The figure shows three views and two pictorial views of one solid part (mm, origin at its lowest corner). Answer the questions. A direction names the side the tool comes from. Coordinates: 2 decimals unless noted, no trailing zeros. Write each loop counter-clockwise with the first axis right and the second up, starting at its lowest first coordinate (ties: lowest second). Pieces come first, ordered by that corner, then holes. Notation, with made-up numbers: M 83.5,6 L 125.5,6 A26 cw 125.5,35 Z; hole C 47.25,63 d2. An arc over 180 degrees is marked long. Answer as CSV lines item,"result".
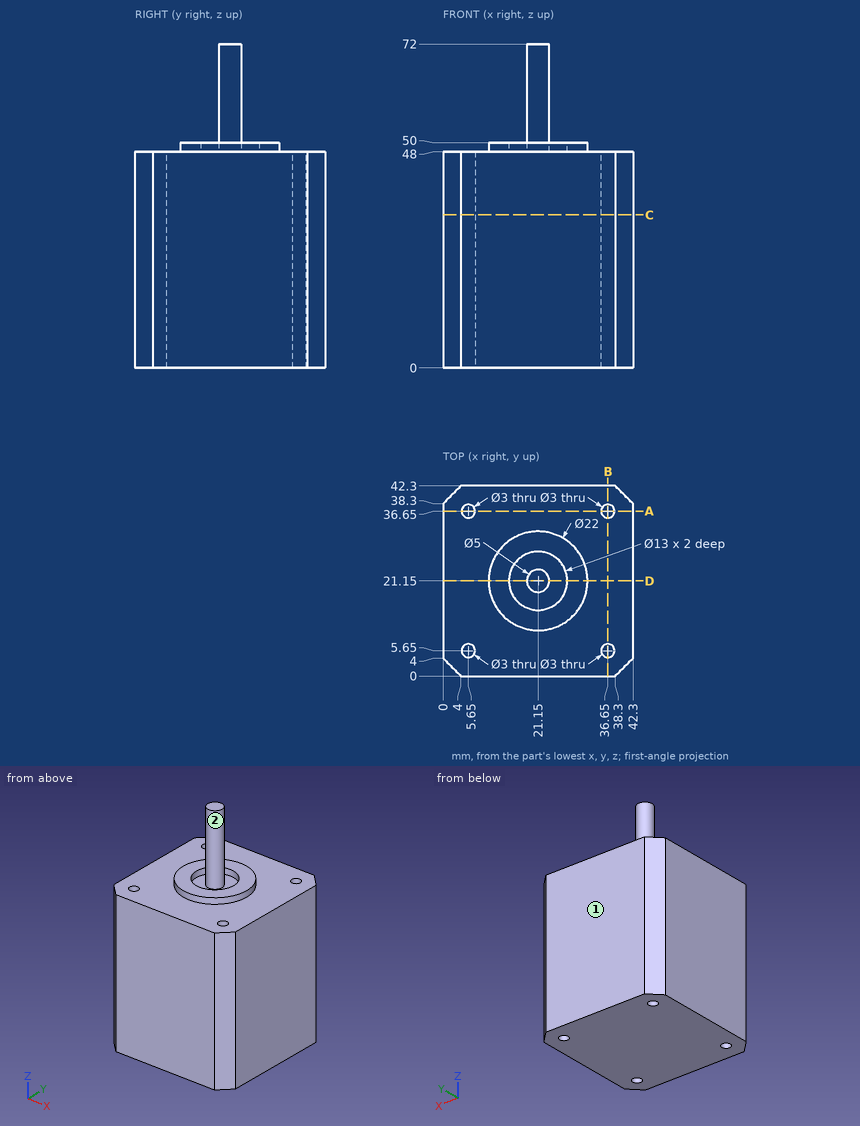
Q1. Find section D-D (y = 21.15). Give the vertices of the cut face in (x, z).
Output:
outline,"M 0,0 L 42.3,0 L 42.3,48 L 32.15,48 L 32.15,50 L 27.65,50 L 27.65,48 L 23.65,48 L 23.65,72 L 18.65,72 L 18.65,48 L 14.65,48 L 14.65,50 L 10.15,50 L 10.15,48 L 0,48 Z"
Q2. Straight lines are drawn through the part: line 1 (Y direction, x = 21.15, z = 49); line 2 (Y direction, x = 5.65, z = 11); line 3 (X direction, y = 5, z = 24). For each, find the intervals that lie inside material, in ascending order.
Output:
line 1,"10.15 to 14.65, 18.65 to 23.65, 27.65 to 32.15"
line 2,"0 to 4.15, 7.15 to 35.15, 38.15 to 42.3"
line 3,"0 to 4.3, 7 to 35.3, 38 to 42.3"
Q3. Find section C-C (z = 34). Give the vertices of the cut face in (x, y), and give its area (3 significant figures).
Output:
outline,"M 0,4 L 4,0 L 38.3,0 L 42.3,4 L 42.3,38.3 L 38.3,42.3 L 4,42.3 L 0,38.3 Z; hole C 5.65,5.65 d3; hole C 5.65,36.65 d3; hole C 36.65,5.65 d3; hole C 36.65,36.65 d3"
area,"1,730 mm2"
Q4. Find section A-A (y = 36.65). Give the vertices of the cut face in (x, z).
Output:
outline,"M 0,0 L 4.15,0 L 4.15,48 L 0,48 Z; M 7.15,0 L 35.15,0 L 35.15,48 L 7.15,48 Z; M 38.15,0 L 42.3,0 L 42.3,48 L 38.15,48 Z"
Q5. For the marked faces 1 and 2, determine the directions among +Z, -Z, +X, -X, +Y, -Y from which every point of the face is accessible in a straight line to the end or side of a thin tool.
Output:
face 1,"+Z, -Z, +X, -X, +Y"
face 2,"+Z"
Q6. Flat-ended cylindrical pins translate along their axes: pin 1 Ø12 at (x, z) = (5, 51) entering from -Y; pin 2 Ø4 at (x, y) = (36.65, 5.65) entering from +Z; pin 3 Ø12.5 at (x, y) = (13, 16) entering from +Z. Find the tip coordinate at first contact, or state that the pin passes through.
Output:
pin 1,"y = 0"
pin 2,"z = 48"
pin 3,"z = 50"
